from build123d import *

# Parameters (mm, degrees)
SKETCH_1_W      = 15
SKETCH_1_H      = 5
SKETCH_1_W_2    = 2
SKETCH_1_H_2    = 2
EXTRUDE_1_DEPTH = 10
SKETCH_1_3_W    = 2
SKETCH_1_3_H    = 2
EXTRUDE_2_DEPTH = 15


with BuildPart() as part:
    # Sketch 1 → Extrude 1 (new body)
    # profile 1 of 4: a face of its own
    with BuildSketch(Plane.XY):
        Rectangle(SKETCH_1_W, SKETCH_1_H)
        Rectangle(SKETCH_1_W_2, SKETCH_1_H_2, mode=Mode.SUBTRACT)
        with Locations((4, 0)):
            Rectangle(SKETCH_1_W_2, SKETCH_1_H_2, mode=Mode.SUBTRACT)
        with Locations((-4, 0)):
            Rectangle(SKETCH_1_W_2, SKETCH_1_H_2, mode=Mode.SUBTRACT)
    # profile 2 of 4: a face of its own
    with BuildSketch(Plane.XY):
        with Locations((4, 0)):
            Rectangle(SKETCH_1_W_2, SKETCH_1_H_2)
    # profile 3 of 4: a face of its own
    with BuildSketch(Plane.XY):
        Rectangle(SKETCH_1_W_2, SKETCH_1_H_2)
    # profile 4 of 4: a face of its own
    with BuildSketch(Plane.XY):
        with Locations((-4, 0)):
            Rectangle(SKETCH_1_W_2, SKETCH_1_H_2)
    extrude(amount=EXTRUDE_1_DEPTH)

    # Sketch 1_3 → Extrude 2 (add)
    with BuildSketch(Plane.XY):
        with Locations((-4, 0)):
            Rectangle(SKETCH_1_3_W, SKETCH_1_3_H)
        Rectangle(SKETCH_1_3_W, SKETCH_1_3_H)
        with Locations((4, 0)):
            Rectangle(SKETCH_1_3_W, SKETCH_1_3_H)
    extrude(amount=EXTRUDE_2_DEPTH)


solid = part.part
Design review of the part built by this model. Coordinates are the model's own, in mm. A direction names the side the tool comes from. Coordinates: 2 decimals unless noted, no trailing zeros. Order: outer loops, then holes, each group sorted by start corner. A loop starts at its lowest first (then second) coordinate and runs counter-clockwise, first axis right, second up. Notation, with made-up numbers: M 54.5,89.5 L 82.5,89.5 A25 ccw 82.5,118.5 Z; hole C 12,86 d7. An arc over 180 degrees is marked long. Use a Markdown table: item, result.
(1) For P1, Ø1, axis at y = 0, z = 13, coming from the -X side; P2, Ø1.6, axis at x = 0, z = 12, coming from the -Y side; P3, Ø3, axis at x = -2.5, z = 12, coming from the +Y side, all flat-tipped, find the tip position at first contact; note any pin that passes through.
Worked answers:
| item | result |
|---|---|
| P1 | stops at x = -5 |
| P2 | stops at y = -1 |
| P3 | stops at y = 1 |
(2) Add section A-A (z = 12.5). Give the boundary of the cut face in (x, y), then the cut area to 3 significant figures.
Worked answers:
| item | result |
|---|---|
| outline | M -5,-1 L -3,-1 L -3,1 L -5,1 Z; M -1,-1 L 1,-1 L 1,1 L -1,1 Z; M 3,-1 L 5,-1 L 5,1 L 3,1 Z |
| area | 12.0 mm2 |
(3) Wall thickness on probe 1 along Z at (x, y) = (-3.75, -1.7); probe 2 along Y at (x, z) = (3.25, 11.5): over which ranges is each line inside the solid? List them lowest first.
Worked answers:
| item | result |
|---|---|
| probe 1 | z = 0 to 10 |
| probe 2 | y = -1 to 1 |
(4) For faces 1 (the flat face through (-4, 1, 12)), 2 (the flat face through (4, -1, 12)), 3 (the flat face through (-1, 0, 12)), list the 3-axis set-ups (+Z, -Z, +X, -X, +Y, -Y) from which the entire face can be reached by the end or side of a thin tool; tool diameter is ignored.
Worked answers:
| item | result |
|---|---|
| face 1 | +Z, +X, -X, +Y |
| face 2 | +Z, +X, -X, -Y |
| face 3 | +Z, +Y, -Y |
(5) Draft analysis for pull direction X (two halves, no side actions). For faces 4 (the flat face through (-4, 0, 15)), 5 (the flat face through (-3, 0, 12)), 6 (the flat face through (1, 0, 12)), 7 (the flat face through (-7.5, 0, 5)), state which applies: released by +X, released by -X, zero draft, split by the parting line, or undercut.
Worked answers:
| item | result |
|---|---|
| face 4 | zero draft |
| face 5 | undercut |
| face 6 | undercut |
| face 7 | released by -X |
(6) Add section C-C (x = 3.5). Give the boundary of the cut face in (y, z), then the cut area to 3 significant figures.
Worked answers:
| item | result |
|---|---|
| outline | M -2.5,0 L 2.5,0 L 2.5,10 L 1,10 L 1,15 L -1,15 L -1,10 L -2.5,10 Z |
| area | 60.0 mm2 |
(7) Add section B-B (y = 0.1). Give the boundary of the cut face in (x, z), then the cut area to 3 significant figures.
Worked answers:
| item | result |
|---|---|
| outline | M -7.5,0 L 7.5,0 L 7.5,10 L 5,10 L 5,15 L 3,15 L 3,10 L 1,10 L 1,15 L -1,15 L -1,10 L -3,10 L -3,15 L -5,15 L -5,10 L -7.5,10 Z |
| area | 180 mm2 |
(8) Add section D-D (y = 1.4). Give the boundary of the cut face in (x, z).
Worked answers:
| item | result |
|---|---|
| outline | M -7.5,0 L 7.5,0 L 7.5,10 L -7.5,10 Z |
